Design review of the part built by this model. Coordinates are the model's own, in mm. A direction names the side the tool comes from. Coordinates: 2 decimals unless noted, no trailing zeros. Order: outer loops, then holes, each group sorted by start corner. A loop starts at its lowest first (then second) coordinate and runs counter-clockwise, first axis right, second up. Notation, with made-up numbers: M -11.75,-24.75 L 31.25,-24.75 A13 cw 31.25,-20.75 Z; hole C 70,78.5 d5. An arc over 180 degrees is marked long. Use CSV: the item, a comma, the result in double quotes.
```python
from build123d import *

# Parameters (mm, degrees)
SKETCH_1_R          = 33.5
SKETCH_1_R_2        = 2.15
SKETCH_1_R_3        = 10
EXTRUDE_1_DEPTH     = 9.9
SKETCH_2_R          = 5
CUT_EXTRUDE_3_DEPTH = 2.5
SKETCH_5_R          = 5
CUT_EXTRUDE_5_DEPTH = 2


with BuildPart() as part:
    # 草图1 → 凸台-拉伸1 (new body)
    with BuildSketch(Plane(origin=(0, 0, 0), x_dir=(1, 0, 0), z_dir=(0, 1, 0))):
        with Locations(Location((0, 0, 0), (0, 0, 90))):
            Circle(SKETCH_1_R)
        with Locations(Location((8.625, 14.938938215, 0), (0, 0, 90))):
            Circle(SKETCH_1_R_2, mode=Mode.SUBTRACT)
        with Locations(Location((0, 0, 0), (0, 0, 90))):
            Circle(SKETCH_1_R_3, mode=Mode.SUBTRACT)
        with Locations(Location((17.25, 0, 0), (0, 0, 90))):
            Circle(SKETCH_1_R_2, mode=Mode.SUBTRACT)
        with Locations(Location((8.625, -14.938938215, 0), (0, 0, 90))):
            Circle(SKETCH_1_R_2, mode=Mode.SUBTRACT)
        with Locations(Location((-8.625, -14.938938215, 0), (0, 0, 90))):
            Circle(SKETCH_1_R_2, mode=Mode.SUBTRACT)
        with Locations(Location((-17.25, 0, 0), (0, 0, 90))):
            Circle(SKETCH_1_R_2, mode=Mode.SUBTRACT)
        with Locations(Location((-8.625, 14.938938215, 0), (0, 0, 90))):
            Circle(SKETCH_1_R_2, mode=Mode.SUBTRACT)
    extrude(amount=EXTRUDE_1_DEPTH)

    # 草图2 → 切除-拉伸3 (cut)
    with BuildSketch(Plane(origin=(0, 0, 0), x_dir=(1, 0, 0), z_dir=(0, 1, 0))):
        with Locations(Location((0, -27, 0), (0, 0, 90))):
            Circle(SKETCH_2_R)
    extrude(amount=CUT_EXTRUDE_3_DEPTH, mode=Mode.SUBTRACT)

    # 草图5 → 切除-拉伸5 (cut)
    with BuildSketch(Plane.XZ):
        with Locations(Location((8.625, 14.938938215, 0), (0, 0, 270))):
            Circle(SKETCH_5_R)
        with Locations(Location((17.25, 0, 0), (0, 0, 270))):
            Circle(SKETCH_5_R)
        with Locations(Location((8.625, -14.938938215, 0), (0, 0, 270))):
            Circle(SKETCH_5_R)
    extrude(amount=-CUT_EXTRUDE_5_DEPTH, mode=Mode.SUBTRACT)


solid = part.part
```
(1) Wall thickness on probe 1 along X at (y, z) = (4, 0); probe 2 along Z at (x, y) = (6.5, 1); probe 3 along Z at (x, y) = (-9, 4.5): over which ranges is each line inside the solid? List them lowest first.
The answers:
probe 1,"x = -33.5 to -19.4, -15.1 to -10, 10 to 15.1, 19.4 to 33.5"
probe 2,"z = -32.86 to -19.46, -10.41 to -7.6, 7.6 to 10.41, 19.46 to 32.86"
probe 3,"z = -32.27 to -17.06, -12.82 to -4.36, 4.36 to 12.82, 17.06 to 32.27"
(2) For faces 4 (the face through (7.98, 5.89, -16.99)), 5 (the face through (12.37, 0.99, 1.08)), list the 3-axis set-ups (+Z, -Z, +X, -X, +Y, -Y) from which the entire face can be reached by the end or side of a thin tool; tool diameter is ignored.
The answers:
face 4,"+Y, -Y"
face 5,"-Y"
(3) Add section B-B on x = 0. State the section outline as (y, z) points.
The answers:
outline,"M 0,-33.5 L 9.9,-33.5 L 9.9,-10 L 0,-10 Z; M 0,10 L 9.9,10 L 9.9,33.5 L 0,33.5 L 0,32 L 2.5,32 L 2.5,22 L 0,22 Z"
(4) Clearance check with flat-ended pins moving along their axes: P1, Ø2.5, axis at x = 8.62, z = 14.94, coming from the +Y side; P2, Ø1, axis at x = 18.5, y = 5.5, coming from the +Z side; P3, Ø6, axis at x = 17.25, z = 0, coming from the -Y side; P4, Ø1, axis at x = 4, y = 5.5, coming from the +Z side. State where each tip first meets the part, or that it passes through.
The answers:
P1,"passes through"
P2,"stops at z = 28.25"
P3,"stops at y = 2"
P4,"stops at z = 33.32"
(5) The part is to be moulded in two halves that separate along Z. For faces 1 (the face through (7, 9.9, 8)), 2 (the face through (9.76, 4.88, 2.17)), 3 (the face through (29.7, 4.9, -15.5)), say which applies: pulls with the +Z half, pulls with the -Z half, needs draft (parallel to the pull), parting line crosses it, or undercut.
The answers:
face 1,"needs draft"
face 2,"undercut"
face 3,"parting line crosses it"
(6) Add section C-C on y = 5. State the section outline as (x, z) points (3 decimals).
The answers:
outline,"C 0,0 d67; hole C -17.25,0 d4.3; hole C -8.625,-14.939 d4.3; hole C -8.625,14.939 d4.3; hole C 0,0 d20; hole C 8.625,-14.939 d4.3; hole C 8.625,14.939 d4.3; hole C 17.25,0 d4.3"
(7) Add section A-A on z = 0. State the section outline as (x, y) points.
The answers:
outline,"M -33.5,0 L -19.4,0 L -19.4,9.9 L -33.5,9.9 Z; M -15.1,0 L -10,0 L -10,9.9 L -15.1,9.9 Z; M 10,0 L 12.25,0 L 12.25,2 L 15.1,2 L 15.1,9.9 L 10,9.9 Z; M 19.4,2 L 22.25,2 L 22.25,0 L 33.5,0 L 33.5,9.9 L 19.4,9.9 Z"
(8) Add section D-D on z = -8. State the section outline as (x, y) points, and give its area (3 significant figures).
The answers:
outline,"M -32.53,0 L -6,0 L -6,9.9 L -32.53,9.9 Z; M 6,0 L 32.53,0 L 32.53,9.9 L 6,9.9 Z"
area,"525 mm2"
